from build123d import *

# Parameters (mm, degrees)
F0_W        = 38.1
F0_H        = 19.05
F1_DEPTH    = 25.4
F2_R        = 3.2639
F3_DEPTH    = 25.4
F4_R        = 4.7625
F5_DEPTH    = 25.4
F6_T1_DEPTH = 84.3707478943
F7_W        = 12.7
F7_H        = 22.225
F8_DEPTH    = 38.1
F9_R        = 5.588
F10_SIZE    = 5.08


# Not quite as in the source:
# - a fillet or chamfer that OpenCascade refuses, or shapes differently, is made with other operations: its cross-section is extruded or revolved along the edge and cut away or added


with BuildPart() as f1:
    # F0 (on Top) → F1 (new body)
    with BuildSketch(Plane.XY):
        with Locations((19.05, 9.525)):
            Rectangle(F0_W, F0_H)
    extrude(amount=-F1_DEPTH)

    # F2 (on face) → F3 (cut)
    with BuildSketch(Plane.XY):
        with Locations((7.3534409022, 9.525)):
            Circle(F2_R)
        with Locations((29.0893973289, 9.525)):
            Circle(F2_R)
    extrude(amount=-F3_DEPTH, mode=Mode.SUBTRACT)

    # F4 (on face) → F5 (cut)
    with BuildSketch(Plane.XZ):
        with Locations((19.05, -16.51)):
            Circle(F4_R)
    extrude(amount=-F5_DEPTH, mode=Mode.SUBTRACT)

    # F6: chamfer of 12.7 on 2 edges, made by hand

    # F6_s2 → F6_t1 (cut)
    with BuildSketch(Plane.XZ.offset(-51.7103739472)):
        Polygon((25.4, -25.4), (38.1, -12.7), (38.1, -25.4), align=None)
        Polygon((0, -12.7), (12.7, -25.4), (0, -25.4), align=None)
    extrude(amount=F6_T1_DEPTH, mode=Mode.SUBTRACT)

    # F7 (on Right) → F8 (cut)
    with BuildSketch(Plane.YZ):
        with Locations((9.525, -14.2875)):
            Rectangle(F7_W, F7_H)
    extrude(amount=F8_DEPTH, mode=Mode.SUBTRACT)

    # F9
    f9_edges = [f1.edges().sort_by_distance(p)[0] for p in [
        (0, 17.4625, -12.7),
        (0, 1.5875, -12.7),
        (12.7, 17.4625, -25.4),
        (12.7, 1.5875, -25.4),
        (25.4, 1.5875, -25.4),
        (25.4, 17.4625, -25.4),
        (38.1, 17.4625, -12.7),
        (38.1, 1.5875, -12.7),
    ]]
    fillet(f9_edges, radius=F9_R)

    # F10
    f10_edges = [f1.edges().sort_by_distance(p)[0] for p in [
        (19.05, 19.05, 0),
        (19.05, 0, 0),
    ]]
    chamfer(f10_edges, length=F10_SIZE)


solid = f1.part
CAD build for the part. Positions are in the model's coordinates, mm. A direction names the side the tool comes from. Round coordinates to 2 decimals unless told otherwise and drop trailing zeros. Loops run counter-clockwise (first coordinate to the right, second up) from the corner with the lowest first, then second, coordinate; pieces in that order, holes last.
(1) Two-plate mould, pull along Y, no slides. Class faces 1 (the flat face through (18.78, 2.5, -2.58)), 2 (the flat face through (19, 9, -3.175)), 3 (the flat face through (19, 10, 0)): +Y half, -Y half, draft (parallel to the pull), parting line (faces both ways), or undercut.
(2) Cut at A-A (x = 19.05). State how many separate pieces and enclosed holes the cut face has, plus the area to 3 significant figures.
(3) Which spindle directions (+Z, -Z, +X, -X, +Y, -Y) get a long thin tool onto all of the face, cutting with end or side? Do faces 4 (the flat face through (19, 15.875, -10)), 5 (the flat face through (0, 9, -3)). Say none if no direction does.
(4) Drop flat-ended pins along their axis: pin 1 (10 mm diameter, centred on x = 13, y = 9.5, fed in from -Z) (3 decimals); pin 2 (3 mm diameter, centred on y = 17, z = -20, fed in from -X). Give the stop position or say it passes through.
(5) Cut at B-B (z = -4). Give the cut face in (x, y) (3 decimals).
(6) Wall check: line 1 along Y through (x, z) = (28.5, -22.25) (3 decimals); line 2 along X through (y, z) = (9.25, -1.25); line 3 along Z through (x, y) = (36, 6.5) (3 decimals). Give the ranges that are in metal, low to high.
Findings below:
1. face 1: -Y half
1. face 2: undercut
1. face 3: draft
2. separate pieces: 3
2. enclosed holes: 0
2. area: 115 mm2
3. face 4: -Z, +X, -X
3. face 5: +Z, -Z, -X, +Y, -Y
4. pin 1: stops at z = -3.175
4. pin 2: stops at x = 5.8
5. outline: (0, 1.08) - (38.1, 1.08) - (38.1, 3.175) - (0, 3.175) - close; (0, 15.875) - (38.1, 15.875) - (38.1, 17.97) - (0, 17.97) - close
6. line 1: y = 0 to 3.175, 15.875 to 19.05
6. line 2: x = 0 to 4.1, 10.61 to 25.84, 32.34 to 38.1
6. line 3: z = -3.175 to 0
